Input: dimensioned drawing with shaded views. Units: mm. Origin: part minimum x, y, z. A direction names the side the tool comes from. Give positions to 0.01 mm unless a question says otherwise; leave off trailing zeros. Write each loop counter-clockwise with the first axis right and the second up, starting at its lowest first coordinate (ties: lowest second). Pieces come first, ordered by that corner, then holes. Notation, with made-up numbers: (49.25, -33.5) -> (63.25, -33.5) arc R26 cw to (63.25, 1.5) -> close; hole circle Ø11 at (-24, 48.25). An arc over 180 degrees is marked (long way). Return JSON: item names as keys, results as strings. Group by question number.
Item 1: Line query: line 1 (X direction, y = 126, z = 62.5); line 2 (Y direction, x = 363, z = 59.5); line 3 (X direction, y = 140.5, z = 73.5). Output: solid intervals per line, ascending. Write a range as [from, to].
Item 2: Section B-B, the plane y = 166.5. Return loops of the section in (x, z), then the cut area to 3 significant figures.
Item 3: Pin query (flat end, axial travel): P1, Ø5.5, axis at y = 67, z = 63, coming from the -X side; P2, Ø2, axis at x = 349, y = 70.5, coming from the +Z side; P3, Ø8, axis at x = 12, y = 70, coming from the +Z side. Return the tip coordinate at first contact, or that it passes through.
Item 4: Set-up query: the marked faces 1 and 2. Return all of +Z, -Z, +X, -X, +Y, -Y with unobstructed straight access to the full face (end or side cutting, diameter ignored); none if empty.
Item 5: Section C-C, the plane x = 155.5. Return loops of the section in (y, z), then the cut area to 3 significant figures.
Item 6: Section A-A, the plane z = 19.5. Return loops of the section in (x, y).
Item 7: Mould query, pull axis Y, two halves, no side actions, for the marked faces 3, 4 and 5. Classes: released by +Y, released by -Y, zero draft, split by the parting line, or undercut.
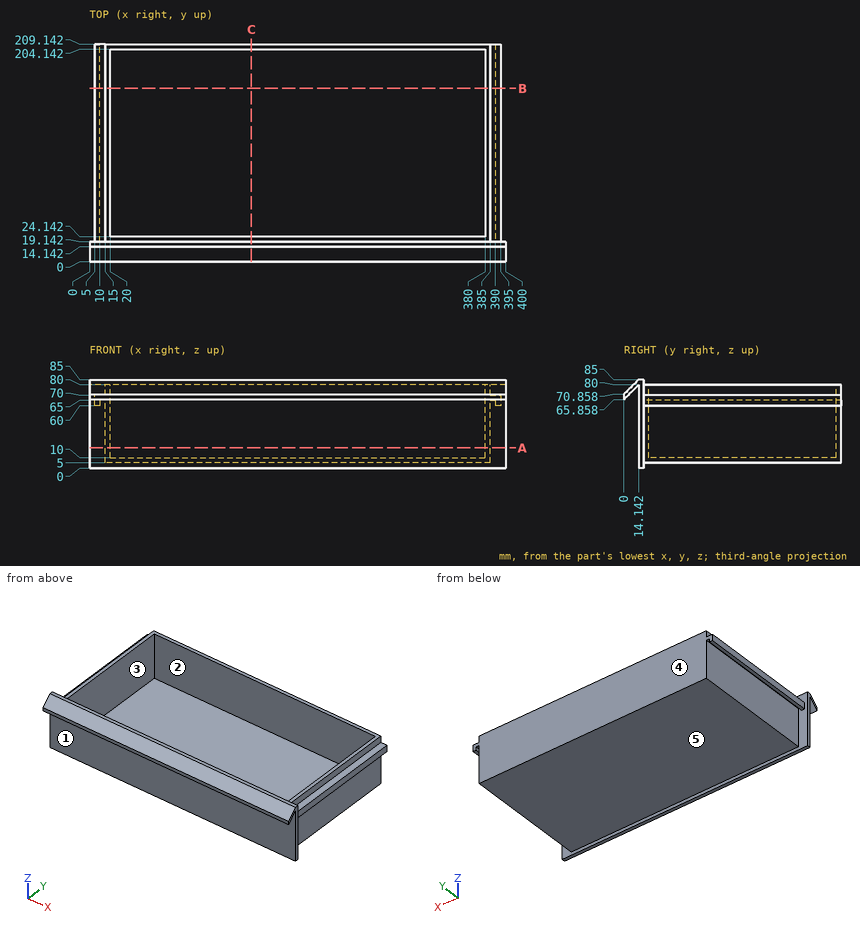
Answer below:
{
 "1": {"line 1": "x = [5, 10], [15, 20], [380, 385], [390, 395]", "line 2": "y = [14.14, 24.14], [204.14, 209.14]", "line 3": "x = [15, 20], [380, 385]"},
 "2": {"outline": "(5, 60) -> (10, 60) -> (10, 65) -> (15, 65) -> (15, 5) -> (385, 5) -> (385, 65) -> (390, 65) -> (390, 60) -> (395, 60) -> (395, 70) -> (385, 70) -> (385, 80) -> (380, 80) -> (380, 10) -> (20, 10) -> (20, 80) -> (15, 80) -> (15, 70) -> (5, 70) -> close", "area": "2,700 mm2"},
 "3": {"P1": "stops at x = 5", "P2": "stops at z = 10", "P3": "stops at z = 80"},
 "4": {"face 1": "-Z, +X, -X", "face 2": "+Z"},
 "5": {"outline": "(0, 65.86) -> (14.14, 80) -> (14.14, 0) -> (19.14, 0) -> (19.14, 5) -> (209.14, 5) -> (209.14, 80) -> (204.14, 80) -> (204.14, 10) -> (24.14, 10) -> (24.14, 80) -> (19.14, 80) -> (19.14, 85) -> (14.14, 85) -> (0, 70.86) -> close", "area": "2,150 mm2"},
 "6": {"outline": "(0, 14.14) -> (400, 14.14) -> (400, 19.14) -> (385, 19.14) -> (385, 209.14) -> (15, 209.14) -> (15, 19.14) -> (0, 19.14) -> close; hole (20, 24.14) -> (380, 24.14) -> (380, 204.14) -> (20, 204.14) -> close"},
 "7": {"face 3": "undercut", "face 4": "released by +Y", "face 5": "zero draft"}
}
